```python
from build123d import *

# Parameters (mm, degrees)
F2_R     = 50.8
F3_R     = 50.8
F4_R     = 2.54
F5_R     = 5.08
F6_DEPTH = 12.7


with BuildPart() as f1:
    # F0 (on Front) → F1 (revolve)
    with BuildSketch(Plane.XZ):
        Polygon((43.18, 63.892171), (38.1, 63.5), (38.1, 31.75), (31.875944, 7.124381), (27.478636, 0), (0, 0), (0, -5.08), (30.312885, -5.08), (36.60948, 5.121546), (43.18, 31.11796), align=None)
    revolve(axis=Axis((0, 0, 31.75), (0, 0, 1)))

    # F2
    f2_edges = [f1.edges().sort_by_distance(p)[0] for p in [
        (-43.18, 0, 31.11796),
        (-36.60948, 0, 5.121546),
    ]]
    fillet(f2_edges, radius=F2_R)

    # F3
    f3_edges = [f1.edges().sort_by_distance(p)[0] for p in [
        (-38.1, 0, 31.75),
        (-31.875944, 0, 7.124381),
    ]]
    fillet(f3_edges, radius=F3_R)

    # F4
    f4_edges = [f1.edges().sort_by_distance(p)[0] for p in [
        (-27.478636, 0, 0),
    ]]
    fillet(f4_edges, radius=F4_R)

    # F5 (on face) → F6 (join)
    with BuildSketch(Plane.XY):
        Circle(F5_R)
    extrude(amount=F6_DEPTH)


solid = f1.part
```
CAD build for the part. Positions are in the model's coordinates, mm. A direction names the side the tool comes from. Give positions to 0.01 mm unless a question says otherwise; leave off trailing zeros. Order: outer loops, then holes, each group sorted by start corner. A loop starts at its lowest first (then second) coordinate and runs counter-clockwise, first axis right, second up. Notation, with made-up numbers: M 32.5,-29.75 L 65.5,-29.75 A19 ccw 65.5,-17.75 Z; hole C -38,9 d4. An arc over 180 degrees is marked long. Put each result on its own line as item: value. Start each with the question number.
(1) Drill centre lines: line 1 along X through (y, z) = (0, 50); line 2 along Z through (x, y) = (23.5, 7). Where is each one in solid material? Low to high.
(2) Saw through at A-A, the plane z = 54.5. Write the cut outline in (x, y), then the cut area to 3 significant figures.
(3) Mould opens along Y. For faces 3 (the flat face through (0, 0, -5.08)), 4 (the cylindrical face through (-30.235, -23.183, 50.607)), 5 (the conical face through (14.051, -27.014, -4.858)) say: +Y half, -Y half, draft (parallel to the pull), parting line (faces both ways), or undercut.
(4) Flat gauge pins, fed straight in: pin 1 Ø5 at (x, z) = (-17.5, 50.5) entering from +Y; pin 2 Ø10 at (y, z) = (-14, 30.5) entering from +X; pin 3 Ø10 at (x, z) = (-3, 10) entering from -Y. Where does each tip first touch, or does it go through?
(5) Which spindle directions (+Z, -Z, +X, -X, +Y, -Y) get a long thin tool onto all of the face, cutting with end or side? Do faces 1 (the flat face through (0, 0, 12.7)), 2 (the cylindrical face through (-31.83, 29.18, 50.85)). Say none if no direction does.
(6) Saw through at B-B, the plane z = 9.5. Give the number of separate pieces and of enclosed holes in the cut face, then the cut area to 3 significant figures.
(7) Saw through at C-C, the plane z = 20. Write the cut outline in (x, y), then the cut area to 3 significant figures.
Check result:
1. line 1: x = -43.18 to -38.1, 38.1 to 43.18
1. line 2: z = -5.08 to 0
2. outline: C 0,0 d86.36; hole C 0,0 d76.2
2. area: 1,300 mm2
3. face 3: draft
3. face 4: undercut
3. face 5: parting line
4. pin 1: stops at y = 40.49
4. pin 2: stops at x = 41.89
4. pin 3: stops at y = -39.03
5. face 1: +Z
5. face 2: +Z, -Z
6. separate pieces: 2
6. enclosed holes: 1
6. area: 1,270 mm2
7. outline: C 0,0 d80.74; hole C 0,0 d70.26
7. area: 1,240 mm2
